Check sheet for the modelled part. Datum: model origin and axes. Units: mm. Round coordinates to 2 decimals unless told otherwise and drop trailing zeros. Write each loop counter-clockwise with the first axis right and the second up, starting at its lowest first coordinate (ties: lowest second). Pieces come first, ordered by that corner, then holes. Notation, with made-up numbers: (-20, 53.25) -> (39, 53.25) arc R25 ccw to (39, 71.25) -> close; hole circle Ø6 at (-33.75, 12). An arc over 180 degrees is marked (long way). Answer as a JSON object with one key per item and string values. Group by question number.
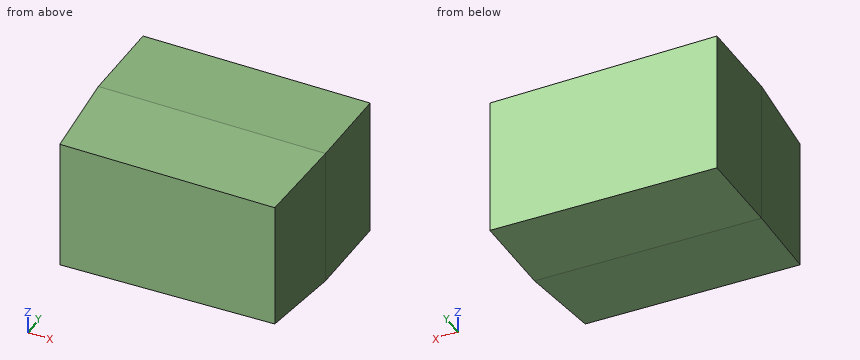
```python
from build123d import *

# Parameters (mm, degrees)
F1_DEPTH      = 25.4
F1_TAPER      = 4
F1_DEPTH_BACK = 25.4


with BuildPart() as f1:
    # F0 (on Front) → F1 (new body, two sides)
    with BuildSketch(Plane.XZ) as f1_sk:
        Polygon((0, 0), (0, -41.8099462986), (66.0554021597, -40.3928682208), (66.0554021597, 0), align=None)
    extrude(amount=F1_DEPTH, taper=F1_TAPER)
    extrude(f1_sk.sketch, amount=-F1_DEPTH_BACK)


solid = f1.part
```
(1) Scan lines: line 1 along X through (y, z) = (-19, -39); line 2 along X through (y, z) = (-12, -38.5); line 3 along Z through (x, y) = (53.5, -8). Record each from-to range of solid material in increasing order.
(2) Go/stop test with flat-tipped pins: pin 1 Ø1 at (x, y) = (27.5, -3.5) entering from -Z; pin 2 Ø1 at (y, z) = (-11, -20) entering from -X; pin 3 Ø3 at (x, y) = (16, -1) entering from -Z. Record where each tip stops, or that it passes through.
(3) Section check A-A on y = 14.5. Record the cut outline in (x, z).
Data:
{
 "1": {"line 1": "x = 1.33 to 64.73", "line 2": "x = 0.84 to 65.22", "line 3": "z = -40.1 to -0.56"},
 "2": {"pin 1": "stops at z = -41.01", "pin 2": "stops at x = 0.73", "pin 3": "stops at z = -41.49"},
 "3": {"outline": "(0, -41.81) -> (66.06, -40.39) -> (66.06, 0) -> (0, 0) -> close"}
}
